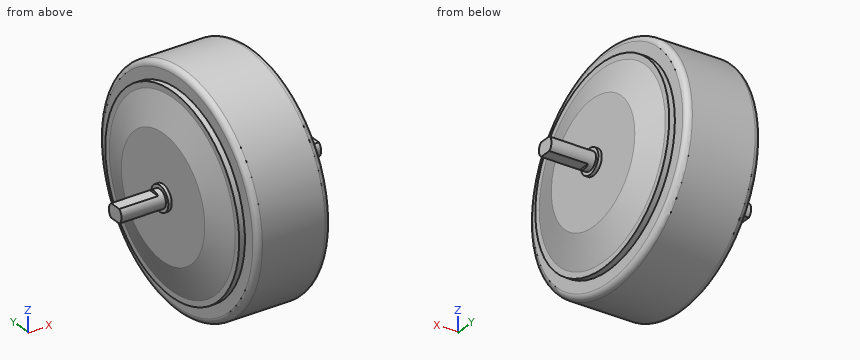
from build123d import *

# Parameters (mm, degrees)
FILLET_1_R           = 5
CUT_EXTRUDE_START    = -53.5
SKETCH_2_OUTSIDE_W   = 268.52
SKETCH_2_OUTSIDE_H   = 268.52
CUT_EXTRUDE_1_DEPTH  = 35
CUT_EXTRUDE_START_2  = 53.5
SKETCH_2_2_OUTSIDE_W = 268.52
SKETCH_2_2_OUTSIDE_H = 268.52
CUT_EXTRUDE_2_DEPTH  = 35


with BuildPart() as part:
    # Эскиз1 → Повернуть1 (revolve)
    with BuildSketch(Plane.XY):
        Polygon((-32.5, 100), (32.5, 100), (32.5, 85), (37.5, 85), (37.5, 80), (45.5, 53), (45.5, 11), (48.5, 11), (48.5, 8), (87.5, 8), (87.5, 0), (-87.5, 0), (-87.5, 8), (-48.5, 8), (-48.5, 11), (-45.5, 11), (-45.5, 53), (-37.5, 80), (-37.5, 85), (-32.5, 85), align=None)
    revolve(axis=Axis((-1100.903674864, 0, 0), (1, 0, 0)))

    # Скругление1
    fillet_1_edges = [part.edges().sort_by_distance(p)[0] for p in [
        (32.5, -100, 0),
        (-32.5, -100, 0),
    ]]
    fillet(fillet_1_edges, radius=FILLET_1_R)

    # Эскиз2 outside → Вырез-Вытянуть1 (cut, through all)
    with BuildSketch(Plane(origin=(0, 0, 0), x_dir=(0, 0, -1), z_dir=(1, 0, 0)).offset(CUT_EXTRUDE_START)):
        Rectangle(SKETCH_2_OUTSIDE_W, SKETCH_2_OUTSIDE_H)
        with BuildLine():
            Line((-6, 5.291502622), (-6, -5.291502622))
            ThreePointArc((-6, -5.291502622), (0, -8), (6, -5.291502622))
            Line((6, -5.291502622), (6, 5.291502622))
            ThreePointArc((6, 5.291502622), (0, 8), (-6, 5.291502622))
        make_face(mode=Mode.SUBTRACT)
    extrude(amount=-CUT_EXTRUDE_1_DEPTH, mode=Mode.SUBTRACT)

    # Эскиз2<2> outside → Вырез-Вытянуть2 (cut, through all)
    with BuildSketch(Plane(origin=(0, 0, 0), x_dir=(0, 0, -1), z_dir=(1, 0, 0)).offset(CUT_EXTRUDE_START_2)):
        Rectangle(SKETCH_2_2_OUTSIDE_W, SKETCH_2_2_OUTSIDE_H)
        with BuildLine():
            Line((-6, 5.291502622), (-6, -5.291502622))
            ThreePointArc((-6, -5.291502622), (0, -8), (6, -5.291502622))
            Line((6, -5.291502622), (6, 5.291502622))
            ThreePointArc((6, 5.291502622), (0, 8), (-6, 5.291502622))
        make_face(mode=Mode.SUBTRACT)
    extrude(amount=CUT_EXTRUDE_2_DEPTH, mode=Mode.SUBTRACT)


solid = part.part
Can you work these out from the model? Positions are in its coordinate system, mm. Round coordinates to 2 decimals unless told otherwise and drop trailing zeros. Write each loop counter-clockwise with the first axis right and the second up, starting at its lowest first coordinate (ties: lowest second). Pieces come first, ordered by that corner, then holes. Notation, with made-up numbers: (53, 42.5) - (67, 42.5) arc R22 ccw to (67, 55.5) - close; hole circle Ø10 at (-36.5, 5.25). An arc over 180 degrees is marked (long way). Write each question's results on one line, items separated by ' | '. Start each with the question number.
1) Suppose I cut it at A-A (x = 59). List the corners of the cut face in (y, z) for me.
2) For pin 1 Ø1.5 at (x, y) = (28, 40) entering from -Z; pin 2 Ø3 at (x, y) = (70.5, 2) entering from -Z; pin 3 Ø1 at (y, z) = (-1.5, -7) entering from -X, each with a flat end and sliding along its axis, tell me the tip position at first contact or that it passes through.
3) Please list where these lines run through material, in increasing order: line 1 (Z direction, x = -23, y = 48.5); line 2 (Y direction, x = 14, z = -60); line 3 (X direction, y = 60.5, z = -61.5).
4) Suppose I cut it at B-B (x = 3). List the corners of the cut face in (y, z) for me.
Here are the results:
1) outline: (-5.29, -6) - (5.29, -6) arc R8 ccw to (5.29, 6) - (-5.29, 6) arc R8 ccw to start
2) pin 1: stops at z = -91.96 | pin 2: stops at z = -6 | pin 3: stops at x = -53.5
3) line 1: z = -87.45 to 87.45 | line 2: y = -80 to 80 | line 3: x = -32.5 to 32.5
4) outline: circle Ø200 at (0, 0)
